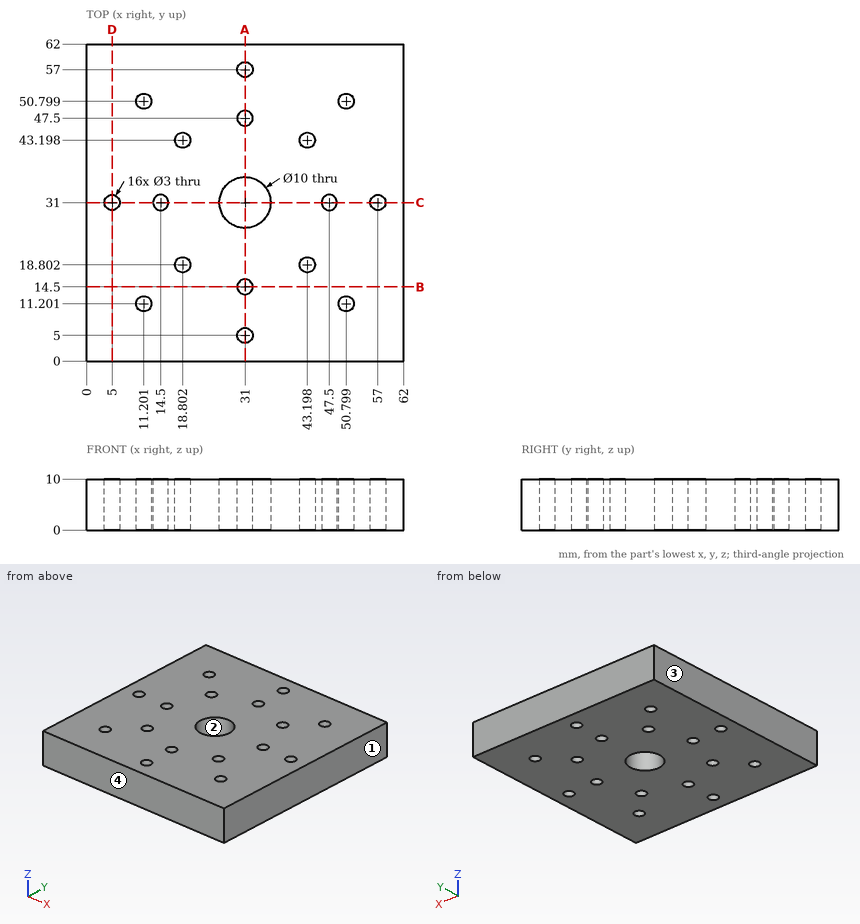
Here's the drawing with two shaded views (mm, measured from the low corner). I have some questions. Give positions to 0.01 mm unless a question says otherwise; leave off trailing zeros. Order: outer loops, then holes, each group sorted by start corner. A loop starts at its lowest first (then second) coordinate and runs counter-clockwise, first axis right, second up. Notation, with made-up numbers: (20.25, 24) -> (28.25, 24) arc R18 cw to (28.25, 48) -> close; hole circle Ø2 at (78, 71.5). An arc over 180 degrees is marked (long way). Use a Markdown table: item, result. Add a question column.
Item 1: Imagine slicing it at A-A on x = 31. Please give me the cut outline in (y, z), plus the area to 3 significant figures.
Item 2: If we mould it in two halves opening along X, with no side actions, what happens to the marked faces 1, 2, 3 and 4? For each: pulls with the +X half, pulls with the -X half, needs draft (parallel to the pull), parting line crosses it, or undercut.
Item 3: Imagine slicing it at B-B on y = 14.5. Please give me the cut outline in (x, z), plus the area to 3 significant figures.
Item 4: I need wall thicknesses on line 1 (Y direction, x = 11, z = 1) (1 decimal); line 2 (Y direction, x = 31, z = 4); line 3 (X direction, y = 43, z = 3) (1 decimal). Which ranges of each line are inside material? Lowest first, please.
Data:
| question | item | result |
|---|---|---|
| 1 | outline | (0, 0) -> (3.5, 0) -> (3.5, 10) -> (0, 10) -> close; (6.5, 0) -> (13, 0) -> (13, 10) -> (6.5, 10) -> close; (16, 0) -> (26, 0) -> (26, 10) -> (16, 10) -> close; (36, 0) -> (46, 0) -> (46, 10) -> (36, 10) -> close; (49, 0) -> (55.5, 0) -> (55.5, 10) -> (49, 10) -> close; (58.5, 0) -> (62, 0) -> (62, 10) -> (58.5, 10) -> close |
| 1 | area | 400 mm² |
| 2 | face 1 | pulls with the +X half |
| 2 | face 2 | undercut |
| 2 | face 3 | pulls with the -X half |
| 2 | face 4 | needs draft |
| 3 | outline | (0, 0) -> (29.5, 0) -> (29.5, 10) -> (0, 10) -> close; (32.5, 0) -> (62, 0) -> (62, 10) -> (32.5, 10) -> close |
| 3 | area | 590 mm² |
| 4 | line 1 | y = 0 to 9.7, 12.7 to 49.3, 52.3 to 62 |
| 4 | line 2 | y = 0 to 3.5, 6.5 to 13, 16 to 26, 36 to 46, 49 to 55.5, 58.5 to 62 |
| 4 | line 3 | x = 0 to 17.3, 20.3 to 41.7, 44.7 to 62 |
